Check sheet for the modelled part. Datum: model origin and axes. Units: mm. Round coordinates to 2 decimals unless told otherwise and drop trailing zeros. Loops run counter-clockwise (first coordinate to the right, second up) from the corner with the lowest first, then second, coordinate; pieces in that order, holes last. Notation, with made-up numbers: (89, -24) - (123, -24) arc R19 cw to (123, 5) - close; hole circle Ø2 at (64, 63.25). An arc over 180 degrees is marked (long way). Return JSON: item names as keys, results as strings.
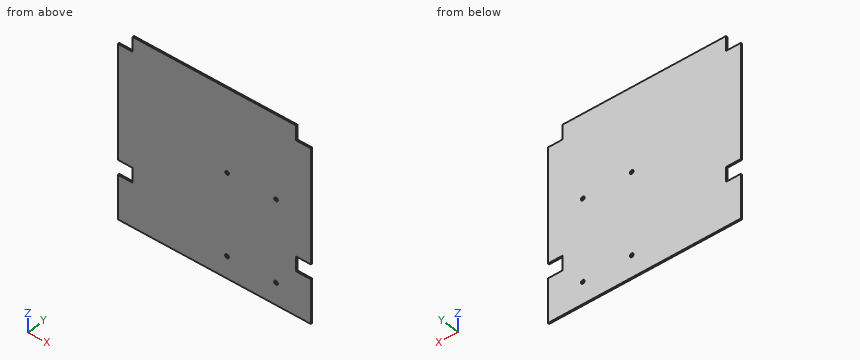
Autodesk Inventor part; units mm, degrees
ref_plane "YZ Plane" through (0, 0, 0) normal (1, 0, 0) x (0, 1, 0)
ref_plane "XZ Plane" through (0, 0, 0) normal (0, 1, 0) x (-1, 0, 0)
ref_plane "XY Plane" through (0, 0, 0) normal (0, 0, 1) x (1, 0, 0)
sketch "Boceto2" plane through (0, 0, 0) normal (0, 1, 0) x (-1, 0, 0)
  line L0 (385.3386, 43.2382) -> (385.3386, -6.7618)
  line L1 (385.3386, -6.7618) -> (435.3386, -6.7618)
  line L2 (385.3386, -446.7618) -> (385.3386, -396.7618)
  line L3 (385.3386, -396.7618) -> (435.3386, -396.7618)
  line L4 (-164.6614, 43.2382) -> (-164.6614, -6.7618)
  line L5 (-164.6614, -6.7618) -> (-214.6614, -6.7618)
  line L6 (-164.6614, -446.7618) -> (-164.6614, -396.7618)
  line L7 (-164.6614, -396.7618) -> (-214.6614, -396.7618)
  line L8 (385.3386, 43.2382) -> (-164.6614, 43.2382)
  line L9 (435.3386, -396.7618) -> (435.3386, -6.7618)
  line L10 (-214.6614, -6.7618) -> (-214.6614, -396.7618)
  line L11 (-164.6614, -446.7618) -> (-214.6614, -446.7618)
  line L12 (-214.6614, -446.7618) -> (-214.6614, -596.7618)
  line L13 (-214.6614, -596.7618) -> (435.3386, -596.7618)
  line L14 (435.3386, -596.7618) -> (435.3386, -446.7618)
  line L15 (435.3386, -446.7618) -> (385.3386, -446.7618)
  point P0 (0, 0)
  dimension "d15" = 50
  dimension "d16" = 50
  dimension "d17" = 50
  dimension "d18" = 50
  dimension "d19" = 50
  dimension "d20" = 50
  dimension "d21" = 50
  dimension "d22" = 50
  dimension "d25" = 50
  dimension "d26" = 150
  dimension "d27" = 650
  dimension "d28" = 150
extrude "Extrusión2" add sketch "Boceto2" along normal blind 5
sketch "Boceto3" plane through (0, 5, 0) normal (0, 1, 0) x (1, 0, 0)
  arc A0 (-61.5546, 521.7618) -> (-74.0546, 521.7618) centre (-67.8046, 521.7618) ccw
  arc A1 (103.4454, 521.7618) -> (90.9454, 521.7618) centre (97.1954, 521.7618) ccw
  arc A2 (90.9454, 241.7618) -> (103.4454, 241.7618) centre (97.1954, 241.7618) ccw
  arc A3 (-74.0546, 241.7618) -> (-61.5546, 241.7618) centre (-67.8046, 241.7618) ccw
  circle A4 centre (-67.8046, 241.7618) radius 6.25
  circle A5 centre (97.1954, 241.7618) radius 6.25
  circle A6 centre (97.1954, 521.7618) radius 6.25
  circle A7 centre (-67.8046, 521.7618) radius 6.25
  point P0 (0, 0)
extrude "Extrusión3" cut sketch "Boceto3" against normal through all
properties material "Aluminio 6061"
Q1. Depth check by flat-ended pin: P1, Ø2.5, axis at x = -411, y = 3.5, coming from the +Z side; P2, Ø2.5, axis at y = 2, z = 19.5, coming from the -X side. Enter the tip coordinate at first touch or a pass-through.
Answer key:
{"P1": "stops at z = -6.76", "P2": "stops at x = -385.34"}
Q2. Sectioned sample at B-B (z = -415). Enter the section's corners in (x, y), plus the area to 3 significant figures.
Answer key:
{"outline": "(-385.34, 0) - (164.66, 0) - (164.66, 5) - (-385.34, 5) - close", "area": "2,750 mm²"}
Q3. Sectioned sample at A-A (y = 2.25). Enter the section's corners in (x, z).
Answer key:
{"outline": "(-435.34, -596.76) - (214.66, -596.76) - (214.66, -446.76) - (164.66, -446.76) - (164.66, -396.76) - (214.66, -396.76) - (214.66, -6.76) - (164.66, -6.76) - (164.66, 43.24) - (-385.34, 43.24) - (-385.34, -6.76) - (-435.34, -6.76) - (-435.34, -396.76) - (-385.34, -396.76) - (-385.34, -446.76) - (-435.34, -446.76) - close; hole circle Ø12.5 at (-67.8, -521.76); hole circle Ø12.5 at (-67.8, -241.76); hole circle Ø12.5 at (97.2, -521.76); hole circle Ø12.5 at (97.2, -241.76)"}
Q4. Scan lines: probe 1 along X at (y, z) = (3.45, -243); probe 2 along Z at (x, y) = (-406, 4.55); probe 3 along X at (y, z) = (4.5, -5). Record each from-to range of solid material in increasing order. Write a range as [from, to].
Answer key:
{"probe 1": "x = [-435.34, -73.93], [-61.68, 91.07], [103.32, 214.66]", "probe 2": "z = [-596.76, -446.76], [-396.76, -6.76]", "probe 3": "x = [-385.34, 164.66]"}
